Solid Edge part; units mm, degrees
sketch "Sketch1" plane through (0, 0, 0) normal (0, -1, 0) x (1, 0, 0)
  line L0 (75, 15) -> (0, 15)
  line L1 (0, 15) -> (0, 0)
  line L2 (0, 0) -> (75, 0)
  line L3 (75, 0) -> (75, 15)
extrude "Protrusion1" add sketch "Sketch1" against normal blind 30
sketch "Sketch2" plane through (37.5, 15, 15) normal (0, 0, 1) x (1, 0, 0)
  line L0 (-22.5, 7.5) -> (22.5, 7.5)
  line L1 (22.5, 7.5) -> (22.5, -7.5)
  line L2 (22.5, -7.5) -> (-22.5, -7.5)
  line L3 (-22.5, -7.5) -> (-22.5, 7.5)
extrude "ExtrudedProtrusion_2" add sketch "Sketch2" along normal blind 90
chamfer "Chamfer_4" distance 22.5 angle 45 1 edges at (60, 15, 105)
chamfer "Chamfer_5" distance 22.5 angle 45 1 edges at (15, 15, 105)
Geometry: final body of the model. Coordinates: model frame, mm. A direction names the side the tool comes from. Round coordinates to 2 decimals unless told otherwise and drop trailing zeros. Order: outer loops, then holes, each group sorted by start corner. A loop starts at its lowest first (then second) coordinate and runs counter-clockwise, first axis right, second up. Notation, with made-up numbers: (-21.75, 69.5) -> (21.25, 69.5) arc R18 cw to (21.25, 75.5) -> close; hole circle Ø1 at (-24.75, 61). An arc over 180 degrees is marked (long way). Put each result on its own line as item: value. Start each with the question number.
Q1. Pull-direction query (Z, two-part tool) for faces 4 (the flat face through (37, 22.5, 59)), 5 (the flat face through (26.1, 15.1, 93.6)), 6 (the flat face through (37, 15, 0)); classes: +Z half, -Z half, draft (parallel to the pull), parting line (faces both ways), or undercut.
Q2. Reachability of faces 1 (the flat face through (38, 7.5, 59)), 2 (the flat face through (15, 15, 48)), 3 (the flat face through (60, 15, 48)) from +Z, -Z, +X, -X, +Y, -Y: full face, straight path, thin tool, end or side. Return the list, or none.
Q3. Section B-B on x = 19.5. Return the cut outline in (y, z).
Q4. Section D-D on x = 35. Return the cut outline in (y, z).
Q5. Line query: probe 1 along Z at (x, y) = (12, 3); probe 2 along X at (y, z) = (19.75, 81); probe 3 along Y at (x, z) = (54.5, 17). Output: solid intervals per line, ascending.
Q6. Section C-C on z = 18.5. Return the cut outline in (x, y).
Q7. First-contact query: pin 1 (3 mm diameter, centred on y = 21, z = 51.5, fed in from -X); pin 2 (8 mm diameter, centred on y = 22, z = 72.5, fed in from +X); pin 3 (12 mm diameter, centred on x = 52.5, z = 41.5, fed in from +Y). Flat tips, straight axial feed; report the tip coordinate or a pass-through.
Ans:
1. face 4: draft
1. face 5: +Z half
1. face 6: -Z half
2. face 1: +Z, +X, -X, -Y
2. face 2: +Z, -X, +Y, -Y
2. face 3: +Z, +X, +Y, -Y
3. outline: (0, 0) -> (30, 0) -> (30, 15) -> (22.5, 15) -> (22.5, 87) -> (7.5, 87) -> (7.5, 15) -> (0, 15) -> close
4. outline: (0, 0) -> (30, 0) -> (30, 15) -> (22.5, 15) -> (22.5, 102.5) -> (7.5, 102.5) -> (7.5, 15) -> (0, 15) -> close
5. probe 1: z = 0 to 15
5. probe 2: x = 15 to 60
5. probe 3: y = 7.5 to 22.5
6. outline: (15, 7.5) -> (60, 7.5) -> (60, 22.5) -> (15, 22.5) -> close
7. pin 1: stops at x = 15
7. pin 2: stops at x = 60
7. pin 3: stops at y = 22.5
